```python
from build123d import *

# Parameters (mm, degrees)
F0_R          = 7.5
F1_DEPTH      = 4
F2_R          = 5
F3_DEPTH      = 100
F4_W          = 4
F4_H          = 4
F5_DEPTH      = 20
F7_DEPTH      = 25
F7_DEPTH_BACK = 25


with BuildPart() as f1:
    # F0 (on Top) → F1 (new body)
    with BuildSketch(Plane.XY):
        Circle(F0_R)
    extrude(amount=F1_DEPTH)

    # F2 (on Top) → F3 (join)
    with BuildSketch(Plane.XY):
        Circle(F2_R)
    extrude(amount=F3_DEPTH)

    # F4 (on face) → F5 (join)
    with BuildSketch(Plane.XY.offset(100)):
        Rectangle(F4_W, F4_H)
    extrude(amount=F5_DEPTH)

    # F6 (on Right) → F7 (cut, two sides)
    with BuildSketch(Plane.YZ) as f7_sk:
        Polygon((0, 121), (-3, 121), (-3, 118), align=None)
    extrude(amount=-F7_DEPTH, mode=Mode.SUBTRACT)
    extrude(f7_sk.sketch, amount=F7_DEPTH_BACK, mode=Mode.SUBTRACT)


solid = f1.part
```
Input: part model. Units: mm. Frame: model coordinates. A direction names the side the tool comes from. Give positions to 0.01 mm unless a question says otherwise; leave off trailing zeros. Write each loop counter-clockwise with the first axis right and the second up, starting at its lowest first coordinate (ties: lowest second). Pieces come first, ordered by that corner, then holes. Notation, with made-up numbers: (47, -38.5) - (99, -38.5) arc R13 ccw to (99, -21.5) - close; hole circle Ø1 at (64, -25). An arc over 180 degrees is marked (long way). Write item = value, one per line. Start each with the question number.
1) Cut plane B-B (x = 0). Return loops of the section in (y, z), and give its area (3 significant figures).
2) Cut plane D-D (z = 108). Return loops of the section in (x, y).
3) Cut plane A-A (y = 0). Return loops of the section in (x, z), and give its area (3 significant figures).
4) Material intervals for L1, parallel to Z at x = 2, y = 4.5; L2, parallel to Z at x = -6.5, y = 0; L3, parallel to X at y = 4.5, z = 56, sorted ascending. Write a range as [from, to].
5) Reachability of faces 1 (the face through (2, -5, 4)), 2 (the face through (-2, 0, 110)), 3 (the face through (0, 2, 110)), 4 (the face through (0, -2, 109)) from +Z, -Z, +X, -X, +Y, -Y: full face, straight path, thin tool, end or side. Return the list, or none.
6) Cut plane C-C (z = 12.5). Return loops of the section in (x, y).
7) Pin query (flat end, axial travel): pin 1 (8 mm diameter, centred on y = -4, z = 51.5, fed in from +X); pin 2 (3 mm diameter, centred on x = 3, y = -3.5, fed in from +Z); pin 3 (6 mm diameter, centred on y = 4, z = 82, fed in from -X). Return the tip coordinate at first contact, or that it passes through.
Answers follow:
q1.outline = (-7.5, 0) - (7.5, 0) - (7.5, 4) - (5, 4) - (5, 100) - (2, 100) - (2, 120) - (-1, 120) - (-2, 119) - (-2, 100) - (-5, 100) - (-5, 4) - (-7.5, 4) - close
q1.area = 1,100 mm^2
q2.outline = (-2, -2) - (2, -2) - (2, 2) - (-2, 2) - close
q3.outline = (-7.5, 0) - (7.5, 0) - (7.5, 4) - (5, 4) - (5, 100) - (2, 100) - (2, 120) - (-2, 120) - (-2, 100) - (-5, 100) - (-5, 4) - (-7.5, 4) - close
q3.area = 1,100 mm^2
q4.L1 = [0, 100]
q4.L2 = [0, 4]
q4.L3 = [-2.18, 2.18]
q5.face_1 = +Z
q5.face_2 = +Z, -X, +Y, -Y
q5.face_3 = +Z, +X, -X, +Y
q5.face_4 = +Z, +X, -X, -Y
q6.outline = circle Ø10 at (0, 0)
q7.pin_1 = 5
q7.pin_2 = 100
q7.pin_3 = -4.9
